from build123d import *

# Parameters (mm, degrees)
SKETCH1_R               = 25.25
SKETCH1_R_2             = 23.25
BOSS_EXTRUDE1_DEPTH     = 210
CUT_EXTRUDE1_REACH      = 215.014
CUT_EXTRUDE1_END_RADIUS = 25.25
SKETCH3_W               = 28
SKETCH3_H               = 122


with BuildPart() as part:
    # Sketch1 → Boss-Extrude1 (new body)
    with BuildSketch(Plane.XY):
        Circle(SKETCH1_R)
        Circle(SKETCH1_R_2, mode=Mode.SUBTRACT)
    extrude(amount=BOSS_EXTRUDE1_DEPTH)

    # Cut-Extrude1: up to this cylinder (the profile starts inside it)
    cut_extrude1_end = Plane(origin=(0, 0, 97), z_dir=(0, 0, -1)) * Cylinder(CUT_EXTRUDE1_END_RADIUS, 481.528, mode=Mode.PRIVATE)
    # Sketch3 → Cut-Extrude1 (cut, up to the surface)
    with BuildSketch(Plane(origin=(0, 0, 0), x_dir=(1, 0, 0), z_dir=(0, 1, 0)), mode=Mode.PRIVATE) as cut_extrude1_sk1:
        with Locations((0, -97)):
            Rectangle(SKETCH3_W, SKETCH3_H)
    cut_extrude1_tool1 = extrude(cut_extrude1_sk1.sketch, amount=-CUT_EXTRUDE1_REACH, mode=Mode.PRIVATE) & cut_extrude1_end
    add(cut_extrude1_tool1.solids().sort_by_distance((0, 0, 97))[0], mode=Mode.SUBTRACT)


solid = part.part
Input: part model. Units: mm. Frame: model coordinates. A direction names the side the tool comes from. Give positions to 0.01 mm unless a question says otherwise; leave off trailing zeros. Loops run counter-clockwise (first coordinate to the right, second up) from the corner with the lowest first, then second, coordinate; pieces in that order, holes last. Notation, with made-up numbers: M -20,19 L 6,19 A37 ccw 6,56 Z; hole C -31.75,62 d5. An arc over 180 degrees is marked long. Use one line per item in the form item = value.
1. Pull-direction query (X, two-part tool) for faces 1 (the face through (22.3, -7.4, 0)), 2 (the face through (-3.287, 25.035, 103.53)), 3 (the face through (-3.03, 23.05, 103.53)); classes: released by +X, released by -X, zero draft, split by the parting line, or undercut.
Numbers:
face_1 = zero draft
face_2 = split by the parting line
face_3 = undercut
2. Line query: L1, parallel to X at y = -1, z = 168; L2, parallel to Y at x = 0, z = 125; L3, parallel to X at y = 6.5, z = 195. Output: solid intervals per line, ascending.
Numbers:
L1 = -25.23 to -23.23, 23.23 to 25.23
L2 = 23.25 to 25.25
L3 = -24.4 to -22.32, 22.32 to 24.4
3. Section query B-B, the plane x = 0. Return the cut outline in (y, z).
Numbers:
outline = M -25.25,0 L -23.25,0 L -23.25,36 L -25.25,36 Z; M -25.25,158 L -23.25,158 L -23.25,210 L -25.25,210 Z; M 23.25,0 L 25.25,0 L 25.25,210 L 23.25,210 Z
4. First-contact query: pin 1 (8 mm diameter, centred on y = -5, z = 67.5, fed in from +X); pin 2 (0.7 mm diameter, centred on y = -19.5, z = 106.5, fed in from -X); pin 3 (1.5 mm diameter, centred on x = 9, z = 116, fed in from +Y); pin 4 (2 mm diameter, centred on x = 3, y = -21, fed in from +Z). Flat tips, straight axial feed; report the tip coordinate or a pass-through.
Numbers:
pin_1 = 25.23
pin_2 = -16.46
pin_3 = 23.86
pin_4 = through
5. Reachability of faces 4 (the face through (22.3, -7.4, 210)), 5 (the face through (-0.1, -23.4, 36)) from +Z, -Z, +X, -X, +Y, -Y: full face, straight path, thin tool, end or side. Return the list, or none.
Numbers:
face_4 = +Z, +X, -X, +Y, -Y
face_5 = -Y
6. Section query D-D, the plane x = 18. Return the cut outline in (y, z).
Numbers:
outline = M -17.71,0 L -14.72,0 L -14.72,210 L -17.71,210 Z; M 14.72,0 L 17.71,0 L 17.71,210 L 14.72,210 Z
7. Section query C-C, the plane z = 189.5. Return the cut outline in (x, y), and give its area (3 significant figures).
Numbers:
outline = C 0,0 d50.5; hole C 0,0 d46.5
area = 305 mm²
8. Section query A-A, the plane y = 0. Return the cut outline in (x, z).
Numbers:
outline = M -25.25,0 L -23.25,0 L -23.25,210 L -25.25,210 Z; M 23.25,0 L 25.25,0 L 25.25,210 L 23.25,210 Z
